from build123d import *

# Parameters (mm, degrees)
F1_DEPTH       = 15
F3_D           = 3.3
F5_D           = 3.3
F5_CSINK_D     = 6.72
F5_CSINK_ANGLE = 90


with BuildPart() as f1:
    # F0 (on Right) → F1 (new body)
    with BuildSketch(Plane.YZ):
        Polygon((0, 15), (0, 0), (15, 0), (15, 2), (2, 2), (2, 15), align=None)
    extrude(amount=F1_DEPTH)

    # F3 (through all)
    with Locations(Plane.XZ):
        with Locations((7.5, 10.5)):
            Hole(F3_D / 2)

    # F5 (through all)
    with Locations(Plane.XY.offset(2)):
        with Locations((7.5, 7.5)):
            CounterSinkHole(F5_D / 2, F5_CSINK_D / 2, counter_sink_angle=F5_CSINK_ANGLE)


solid = f1.part
Design review of the part built by this model. Coordinates are the model's own, in mm. A direction names the side the tool comes from. Coordinates: 2 decimals unless noted, no trailing zeros. Loops run counter-clockwise (first coordinate to the right, second up) from the corner with the lowest first, then second, coordinate; pieces in that order, holes last. Notation, with made-up numbers: (22.5, 34.5) -> (32.5, 34.5) arc R28 ccw to (32.5, 67.5) -> close; hole circle Ø10 at (-1.5, -40). An arc over 180 degrees is marked (long way). Use a Markdown table: item, result. Add a question column.
Item 1: The part is to be moulded in two halves that separate along Z. For faces 3 (the flat face through (7, 2, 8)), 4 (the flat face through (7.4, 5.7, 0)), 5 (the flat face through (7, 1, 15)), 6 (the cylindrical face through (8.81, 1.01, 9.5)), say which applies: +Z half, -Z half, draft (parallel to the pull), parting line (faces both ways), or undercut.
Item 2: We need section D-D, the plane x = 11.25. Write out the cut boundary in (y, z), and give its area (3 significant figures).
Item 3: We need section C-C, the plane y = 7.5. Write out the cut boundary in (x, z).
Item 4: We need section B-B, the plane z = 10.5. Write out the cut boundary in (x, y), and give its area (3 significant figures).
Item 5: We need section A-A, the plane x = 7.5. Write out the cut boundary in (y, z), and give its area (3 significant figures).
Item 6: Wall thickness on L1, parallel to Y at x = 7.5, z = 0.15; L2, parallel to Z at x = 7.5, y = 0.7: over which ranges is each line inside the solid? List them lowest first. Write a range as from..to.
Item 7: Clearance check with a flat-ended pin moving along its axis: P1, Ø4, axis at x = 6, z = 9, coming from the +Y side. State where the tip first meets the part, or that it passes through.
Item 8: Machinability: for faces 1 (the flat face through (15, 1, 5)), 2 (the flat face through (7, 11, 2)), which of the approach directions +Z, -Z, +X, -X, +Y, -Y give a long, thin tool a straight path to every point of the face, cutting with its end or side? Answer none if there is none.
Numbers:
| question | item | result |
|---|---|---|
| 1 | face 3 | draft |
| 1 | face 4 | -Z half |
| 1 | face 5 | +Z half |
| 1 | face 6 | undercut |
| 2 | outline | (0, 0) -> (15, 0) -> (15, 2) -> (2, 2) -> (2, 15) -> (0, 15) -> close |
| 2 | area | 56.0 mm^2 |
| 3 | outline | (0, 0) -> (5.85, 0) -> (5.85, 0.29) -> (4.14, 2) -> (0, 2) -> close; (9.15, 0) -> (15, 0) -> (15, 2) -> (10.86, 2) -> (9.15, 0.29) -> close |
| 4 | outline | (0, 0) -> (5.85, 0) -> (5.85, 2) -> (0, 2) -> close; (9.15, 0) -> (15, 0) -> (15, 2) -> (9.15, 2) -> close |
| 4 | area | 23.4 mm^2 |
| 5 | outline | (0, 0) -> (5.85, 0) -> (5.85, 0.29) -> (4.14, 2) -> (2, 2) -> (2, 8.85) -> (0, 8.85) -> close; (0, 12.15) -> (2, 12.15) -> (2, 15) -> (0, 15) -> close; (9.15, 0) -> (15, 0) -> (15, 2) -> (10.86, 2) -> (9.15, 0.29) -> close |
| 5 | area | 39.9 mm^2 |
| 6 | L1 | y = 0..5.85, 9.15..15 |
| 6 | L2 | z = 0..8.85, 12.15..15 |
| 7 | P1 | stops at y = 2 |
| 8 | face 1 | +Z, -Z, +X, +Y, -Y |
| 8 | face 2 | +Z, +X, -X, +Y |
